Source: CAD feature listing. Evaluate the final solid. Frame: model axes, mm. A direction names the side the tool comes from. Coordinates: 2 decimals unless noted, no trailing zeros. Order: outer loops, then holes, each group sorted by start corner. A loop starts at its lowest first (then second) coordinate and runs counter-clockwise, first axis right, second up.
Item 1: Mould query, pull axis Y, two halves, no side actions, for faces 1 (the flat face through (-12.86, 3.93, 0.99)), 2 (the cylindrical face through (10.621, 0.845, 0.986)), 3 (the flat face through (7.3, 0.2, 0)), 4 (the cylindrical face through (-7.02, 7.12, 0.99)). Classes: released by +Y, released by -Y, zero draft, split by the parting line, or undercut.
Item 2: Section A-A on z = 5.5. Return the cut outline in (x, y), then the cut area to 3 significant figures.
Item 3: Ray query, line 1 (X direction, y = -10.75, z = 5.7); line 2 (X direction, y = -12, z = 2.25); line 3 (Z direction, x = -9, y = 4). Return the intervals inside material, ascending.
Item 4: Reachability of faces 5 (the flat face through (0, -13, 6.5)), 6 (the flat face through (-3.25, -12, 4)), 7 (the cylindrical face through (-6.466, -2.681, 0.986)), 8 (the cylindrical face through (0, 7.5, 4.2)), 9 (the flat face through (3.25, 12, 4)) from +Z, -Z, +X, -X, +Y, -Y: full face, straight path, thin tool, end or side. Return the list, or none.
Item 5: Section C-C on x = 10. Return the cut outline in (y, z), then the cut area to 3 significant figures.
Item 6: Contact query for flat-ended pins moving along their axis: P1, Ø0.9, axis at x = -4, y = 14, coming from the +Z side; P2, Ø2, axis at y = -6.5, z = 4.5, coming from the -X side; P3, Ø1.2, axis at x = -0.5, y = 10.5, coming from the +Z side. Output: stop coordinate, or through.
Item 7: Section D-D on z = 1.5. Return the cut outline in (x, y).
Item 8: Section B-B on y = 0. Return the cut outline in (x, z), then the cut area to 3 significant figures.
from build123d import *

# Parameters (mm, degrees)
SKETCH_1_R          = 17
EXTRUDE_1_DEPTH     = 2
SKETCH_2_R          = 7
CUT_EXTRUDE_1_DEPTH = 2
CUT_EXTRUDE_3_DEPTH = 2.5
EXTRUDE_6_DEPTH     = 4.5
SKETCH_25_R         = 1.25
CUT_EXTRUDE_4_DEPTH = 4
SKETCH_27_R         = 1.25
CUT_EXTRUDE_5_DEPTH = 2


with BuildPart() as part:
    # 草图1 → 凸台-拉伸1 (new body)
    with BuildSketch(Plane.XY):
        Circle(SKETCH_1_R)
    extrude(amount=EXTRUDE_1_DEPTH)

    # 草图2 → 切除-拉伸1 (cut)
    with BuildSketch(Plane(origin=(0, 0, 0), x_dir=(-1, 0, 0), z_dir=(0, 0, -1))):
        Circle(SKETCH_2_R)
    extrude(amount=-CUT_EXTRUDE_1_DEPTH, mode=Mode.SUBTRACT)

    # 草图11 → 切除-拉伸3 (cut)
    with BuildSketch(Plane(origin=(0, 0, 0), x_dir=(-1, 0, 0), z_dir=(0, 0, -1))):
        with BuildLine():
            Line((4.97031898, 16.257180851), (2.923717047, 9.56304756))
            ThreePointArc((2.923717047, 9.56304756), (7.071067812, 7.071067812), (9.56304756, 2.923717047))
            Line((9.56304756, 2.923717047), (16.257180851, 4.97031898))
            ThreePointArc((16.257180851, 4.97031898), (12.02081528, 12.02081528), (4.97031898, 16.257180851))
        make_face()
    extrude(amount=-CUT_EXTRUDE_3_DEPTH, mode=Mode.SUBTRACT)

    # 草图24 → 凸台-拉伸6 (add)
    with BuildSketch(Plane.XY.offset(2)):
        with BuildLine():
            Line((3.25, 16.686446596), (3.25, 6.759252917))
            ThreePointArc((3.25, 6.759252917), (0, 7.5), (-3.25, 6.759252917))
            Line((-3.25, 6.759252917), (-3.25, 16.686446596))
            ThreePointArc((-3.25, 16.686446596), (0, 17), (3.25, 16.686446596))
        make_face()
        with BuildLine():
            Line((3.25, -16.686446596), (3.25, -6.759252917))
            ThreePointArc((3.25, -6.759252917), (0, -7.5), (-3.25, -6.759252917))
            Line((-3.25, -6.759252917), (-3.25, -16.686446596))
            ThreePointArc((-3.25, -16.686446596), (0, -17), (3.25, -16.686446596))
        make_face()
    extrude(amount=EXTRUDE_6_DEPTH)

    # 草图25 → 切除-拉伸4 (cut)
    with BuildSketch(Plane.XY.offset(6.5)):
        with Locations((0, 10.75)):
            Circle(SKETCH_25_R)
        with Locations(Location((0, -10.75, 0), (0, 0, 180))):
            Circle(SKETCH_25_R)
    extrude(amount=-CUT_EXTRUDE_4_DEPTH, mode=Mode.SUBTRACT)

    # 草图27 → 切除-拉伸5 (cut)
    with BuildSketch(Plane(origin=(0, 0, 0), x_dir=(-1, 0, 0), z_dir=(0, 0, -1))):
        with Locations((-9.7, 0)):
            Circle(SKETCH_27_R)
        with Locations((9.7, 0)):
            Circle(SKETCH_27_R)
    extrude(amount=-CUT_EXTRUDE_5_DEPTH, mode=Mode.SUBTRACT)


solid = part.part
Answer list:
1. face 1: released by +Y
1. face 2: undercut
1. face 3: zero draft
1. face 4: undercut
2. outline: (-3.25, -16.69) arc R17 ccw to (3.25, -16.69) - (3.25, -6.76) arc R7.5 cw to (-3.25, -6.76) - close; (-3.25, 6.76) arc R7.5 cw to (3.25, 6.76) - (3.25, 16.69) arc R17 ccw to (-3.25, 16.69) - close; hole circle Ø2.5 at (0, -10.75); hole circle Ø2.5 at (0, 10.75)
2. area: 115 mm2
3. line 1: x = -3.25 to -1.25, 1.25 to 3.25
3. line 2: x = -3.25 to 3.25
3. line 3: z = 0 to 2
4. face 5: +Z, +X, -X, +Y, -Y
4. face 6: +Z, -X, +Y, -Y
4. face 7: +Z, -Z
4. face 8: +Z
4. face 9: +Z, +X, +Y, -Y
5. outline: (-13.75, 0) - (-1.21, 0) - (-1.21, 2) - (-13.75, 2) - close; (1.21, 0) - (13.75, 0) - (13.75, 2) - (1.21, 2) - close
5. area: 50.1 mm2
6. P1: stops at z = 2
6. P2: stops at x = -3.25
6. P3: stops at z = 2.5
7. outline: (-16.26, 4.97) arc R17 ccw (long way) to (-4.97, 16.26) - (-2.92, 9.56) arc R10 ccw to (-9.56, 2.92) - close; hole circle Ø2.5 at (-9.7, 0); hole circle Ø14 at (0, 0); hole circle Ø2.5 at (9.7, 0)
8. outline: (-17, 0) - (-10.95, 0) - (-10.95, 2) - (-17, 2) - close; (-8.45, 0) - (-7, 0) - (-7, 2) - (-8.45, 2) - close; (7, 0) - (8.45, 0) - (8.45, 2) - (7, 2) - close; (10.95, 0) - (17, 0) - (17, 2) - (10.95, 2) - close
8. area: 30.0 mm2
